Geometry check sheet. Reference: the model listing, model coordinates, mm. Face numbers are marked on the shaded views. A direction names the side the tool comes from. Coordinates: 2 decimals unless noted, no trailing zeros. Loops run counter-clockwise (first coordinate to the right, second up) from the corner with the lowest first, then second, coordinate; pieces in that order, holes last. Notation, with made-up numbers: (-7.75, 42.5) - (24.25, 42.5) arc R19 ccw to (24.25, 63.5) - close; hole circle Ø4 at (54.5, 19). An arc over 180 degrees is marked (long way). Write each question's results on one line, items separated by ' | '. Start each with the question number.
(1) Go/stop test with flat-tipped pins: pin 1 Ø8 at (x, z) = (-38, 23.5) entering from +Y; pin 2 Ø8 at (x, z) = (-50, 23.5) entering from +Y; pin 3 Ø10.5 at (x, z) = (-7.98, 43.02) entering from +Y; pin 4 Ø10 at (x, y) = (-30, 4) entering from +Z. Record where each tip stops, or that it passes through.
(2) Material ranges on probe 1 along X at (y, z) = (0.5, 18); probe 2 along X at (y, z) = (3.5, 40.5); probe 3 along X at (y, z) = (2, 29.5), recorded low to high.
(3) Sectioned sample at B-B (z = 42). State how many separate pieces and enclosed holes the cut face has, plus the area to 3 significant figures.
(4) Access from +Z, -Z, +X, -X, +Y, -Y to the whole of each face (thin tool, end or side, straight path). Record for the marked faces 5, 6, 7 and 8.
(5) Sectioned sample at C-C (x = 2.5). Enter the section's corners in (y, z).
(6) Sectioned sample at A-A (z = 18.5). Enter the section's corners in (x, y), plus the area to 3 significant figures.
(7) Mould release check, pull along X, two halves, no side actions. Record for the marked faces 1, 2, 3 and 4: pulls with the +X half, pulls with the -X half, needs draft (parallel to the pull), parting line crosses it, or undercut.
(8) Sectioned sample at D-D (x = -45.5). Enter the section's corners in (y, z).
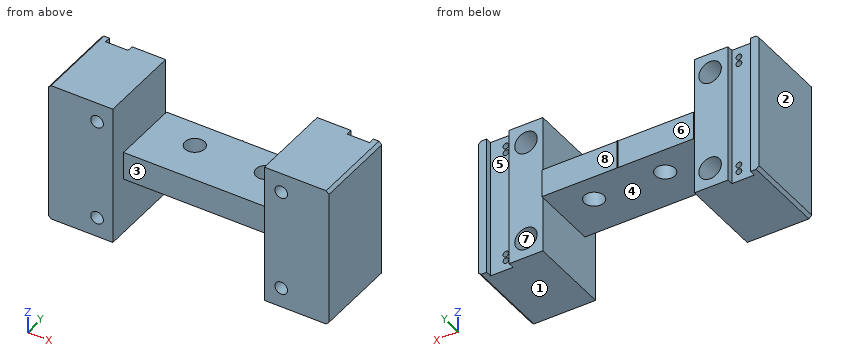
from build123d import *

# Parameters (mm, degrees)
BOSS_EXTRUDE1_DEPTH     = 50
SKETCH2_W               = 10
SKETCH2_H               = 30
BOSS_EXTRUDE2_DEPTH     = 54
BOSS_EXTRUDE4_DEPTH     = 10
BOSS_EXTRUDE5_DEPTH     = 50
SKETCH5_R               = 3.5
CUT_EXTRUDE1_DEPTH      = 54
SKETCH6_R               = 2.25
CUT_EXTRUDE2_DEPTH      = 30.5
SKETCH7_R               = 4
CUT_EXTRUDE3_DEPTH      = 10
M2_5_TAPPED_HOLE2_D     = 2.05
M2_5_TAPPED_HOLE2_DEPTH = 6.35
M2_5_TAPPED_HOLE2_TIP   = 0.615882135
CHAMFER1_SIZE           = 1
SKETCH14_W              = 54
SKETCH14_H              = 6
CUT_EXTRUDE4_DEPTH      = 10


with BuildPart() as part:
    # Sketch1 → Boss-Extrude1 (new body)
    with BuildSketch(Plane.XY):
        Polygon((6.013513514, 8.114864865), (9.013513514, 8.114864865), (9.013513514, -21.385135135), (-13.986486486, -21.385135135), (-13.986486486, 8.114864865), (-1.986486486, 8.114864865), (-1.986486486, 5.964864865), (6.013513514, 5.964864865), align=None)
    extrude(amount=BOSS_EXTRUDE1_DEPTH)

    # Sketch2 → Boss-Extrude2 (add)
    with BuildSketch(Plane.ZY.offset(13.986486486)):
        with Locations((25, -6.385135135)):
            Rectangle(SKETCH2_W, SKETCH2_H)
    extrude(amount=BOSS_EXTRUDE2_DEPTH)

    # Sketch3 → Boss-Extrude4 (add)
    with BuildSketch(Plane(origin=(0, 0, 20), x_dir=(-1, 0, 0), z_dir=(0, 0, -1))):
        Polygon((40.811486486, 8.614864865), (40.986486486, 8.917973756), (41.161486486, 8.614864865), align=None)
    extrude(amount=-BOSS_EXTRUDE4_DEPTH)

    # Sketch4 → Boss-Extrude5 (add)
    with BuildSketch(Plane(origin=(0, 0, 0), x_dir=(-1, 0, 0), z_dir=(0, 0, -1))):
        Polygon((67.986486486, 8.114864865), (79.986486486, 8.114864865), (79.986486486, 5.964864865), (87.986486486, 5.964864865), (87.986486486, 8.114864865), (90.986486486, 8.114864865), (90.986486486, -21.385135135), (67.986486486, -21.385135135), align=None)
    extrude(amount=-BOSS_EXTRUDE5_DEPTH)

    # Sketch5 → Cut-Extrude1 (cut)
    with BuildSketch(Plane(origin=(0, 0, 20), x_dir=(-1, 0, 0), z_dir=(0, 0, -1))):
        with Locations((26.537216594, -0.885135135)):
            Circle(SKETCH5_R)
        with Locations((51.838124653, -0.885135135)):
            Circle(SKETCH5_R)
    extrude(amount=-CUT_EXTRUDE1_DEPTH, mode=Mode.SUBTRACT)

    # Sketch6 → Cut-Extrude2 (cut, through all)
    with BuildSketch(Plane(origin=(0, 8.114864865, 0), x_dir=(1, 0, 0), z_dir=(0, 1, 0))):
        with Locations((-7.981926448, -7.026366578)):
            Circle(SKETCH6_R)
        with Locations((-7.981926448, -43.021631087)):
            Circle(SKETCH6_R)
        with Locations((-73.593710074, -43.021631087)):
            Circle(SKETCH6_R)
        with Locations((-73.593710074, -7.026366578)):
            Circle(SKETCH6_R)
    extrude(amount=-CUT_EXTRUDE2_DEPTH, mode=Mode.SUBTRACT)

    # Sketch7 → Cut-Extrude3 (cut)
    with BuildSketch(Plane(origin=(0, 8.114864865, 0), x_dir=(1, 0, 0), z_dir=(0, 1, 0))):
        with Locations((-7.981926448, -43.021631087)):
            Circle(SKETCH7_R)
        with Locations((-7.981926448, -7.026366578)):
            Circle(SKETCH7_R)
        with Locations((-73.593710074, -43.021631087)):
            Circle(SKETCH7_R)
        with Locations((-73.593710074, -7.026366578)):
            Circle(SKETCH7_R)
    extrude(amount=-CUT_EXTRUDE3_DEPTH, mode=Mode.SUBTRACT)

    # M2.5 Tapped Hole2
    with Locations(Plane(origin=(0, 5.964864865, 0), x_dir=(1, 0, 0), z_dir=(0, 1, 0))):
        with Locations((0.513513514, -46.5), (0.513513514, -3.5), (-82.486486486, -46.5), (-82.486486486, -3.5), (0.513513514, -44), (0.513513514, -6), (-82.486486486, -44), (-82.486486486, -6)):
            Hole(M2_5_TAPPED_HOLE2_D / 2, depth=M2_5_TAPPED_HOLE2_DEPTH)
            with Locations((0, 0, -(M2_5_TAPPED_HOLE2_DEPTH + M2_5_TAPPED_HOLE2_TIP / 2))):  # 118° drill point
                Cone(0, M2_5_TAPPED_HOLE2_D / 2, M2_5_TAPPED_HOLE2_TIP, mode=Mode.SUBTRACT)

    # Chamfer1
    chamfer1_edges = [part.edges().sort_by_distance(p)[0] for p in [
        (9.013513514, -6.635135135, 50),
        (-90.986486486, -6.635135135, 50),
        (-90.986486486, -6.635135135, 0),
        (9.013513514, -6.635135135, 0),
    ]]
    chamfer(chamfer1_edges, length=CHAMFER1_SIZE)

    # Sketch14 → Cut-Extrude4 (cut)
    with BuildSketch(Plane(origin=(0, 0, 20), x_dir=(-1, 0, 0), z_dir=(0, 0, -1))):
        with Locations((40.986486486, -18.385135135)):
            Rectangle(SKETCH14_W, SKETCH14_H)
    extrude(amount=-CUT_EXTRUDE4_DEPTH, mode=Mode.SUBTRACT)


solid = part.part
Outcome:
1) pin 1: stops at y = 8.92 | pin 2: stops at y = 8.61 | pin 3: stops at y = 8.11 | pin 4: stops at z = 30
2) probe 1: x = -90.99 to -67.99, -13.99 to 9.01 | probe 2: x = -90.99 to -76.7, -70.49 to -67.99, -13.99 to -11.09, -4.88 to 9.01 | probe 3: x = -90.99 to -53.82, -49.86 to -28.52, -24.56 to 9.01
3) separate pieces: 4 | enclosed holes: 0 | area: 1,010 mm2
4) face 5: +Z, -Z, +Y | face 6: +Z, -Z, -X, +Y | face 7: +Y | face 8: +Z, -Z, +X, +Y
5) outline: (-21.39, 0) - (5.96, 0) - (5.96, 50) - (-21.39, 50) - close
6) outline: (-90.99, -21.39) - (-67.99, -21.39) - (-67.99, 8.11) - (-79.99, 8.11) - (-79.99, 5.96) - (-87.99, 5.96) - (-87.99, 8.11) - (-90.99, 8.11) - close; (-13.99, -21.39) - (9.01, -21.39) - (9.01, 8.11) - (6.01, 8.11) - (6.01, 5.96) - (-1.99, 5.96) - (-1.99, 8.11) - (-13.99, 8.11) - close | area: 1,320 mm2
7) face 1: needs draft | face 2: pulls with the -X half | face 3: undercut | face 4: undercut
8) outline: (-15.39, 20) - (8.61, 20) - (8.61, 30) - (-15.39, 30) - close
